from build123d import *

# Parameters (mm, degrees)
F0_R     = 8.25
F1_DEPTH = 2.5
F2_DEPTH = 2


with BuildPart() as f1:
    # F0 (on Top) → F1 (new body)
    with BuildSketch(Plane.XY):
        with BuildLine():
            ThreePointArc((32.0688115177, 8.9962420553), (27.6273312583, -1.0959733646), (33.9415177003, -10.1353654102))
            ThreePointArc((33.9415177003, -10.1353654102), (44.8086587224, -9.5259748044), (50.073819207, 0))
            ThreePointArc((50.073819207, 0), (43.8521719937, 10.0637054931), (32.0688115177, 8.9962420553))
        make_face()
        with Locations((38.823819207, 0)):
            Circle(F0_R, mode=Mode.SUBTRACT)
    extrude(amount=F1_DEPTH)



with BuildPart() as f1b:
    # F0 (on Top) → F1, piece 2 (new body)
    with BuildSketch(Plane.XY):
        with BuildLine():
            ThreePointArc((-45.6604546957, -2.0769858561), (-38.7231383621, 8.1832988366), (-29.426180793, 0))
            ThreePointArc((-29.426180793, 0), (-29.8634270645, -2.6501658772), (-31.1288181692, -5.0194165669))
            ThreePointArc((-31.1288181692, -5.0194165669), (-31.2694247122, -5.1976895367), (-31.4148838182, -5.3720257066))
            add(Edge.make_bspline(
                [(-29.035736161, -7.2045275043), (-30.5396230029, -7.95646964), (-32.2793337143, -6.7201835537), (-31.4148838182, -5.3720257066)],
                knots=[0, 0, 0, 0, 2.7840168374, 2.7840168374, 2.7840168374, 2.7840168374], degree=3))
            ThreePointArc((-29.035736161, -7.2045275043), (-27.0986692211, -3.8312855473), (-26.426180793, 0))
            ThreePointArc((-26.426180793, 0), (-27.6571196172, 5.1167287553), (-31.080565354, 9.1137454968))
            ThreePointArc((-31.080565354, 9.1137454968), (-44.3248746058, 9.0750961749), (-48.354220505, -3.5414640914))
            add(Edge.make_bspline(
                [(-45.6604546957, -2.0769858561), (-46.4311366211, -5.0662274962), (-47.7208728718, -5.0662274962), (-48.354220505, -3.5414640914)],
                knots=[0, 0, 0, 0, 3.0661165562, 3.0661165562, 3.0661165562, 3.0661165562], degree=3))
        make_face()
    extrude(amount=F1_DEPTH)


with BuildPart() as f1_1:
    add(f1.part)

    add(f1b.part)  # F2 merges F1b
    # F0 (on Top) → F2 (join)
    with BuildSketch(Plane.XY):
        with BuildLine():
            ThreePointArc((-26.426180793, 0), (-27.0986692211, -3.8312855473), (-29.035736161, -7.2045275043))
            add(Edge.make_bspline(
                [(-29.035736161, -7.2045275043), (-3.4389084727, 0), (5.4949232749, 0), (33.9415177003, -10.1353654102)],
                knots=[0, 0, 0, 0, 63.0454147004, 63.0454147004, 63.0454147004, 63.0454147004], degree=3))
            ThreePointArc((33.9415177003, -10.1353654102), (27.6273312583, -1.0959733646), (32.0688115177, 8.9962420553))
            add(Edge.make_bspline(
                [(-31.080565354, 9.1137454968), (-3.4389084727, 0), (5.4949232749, 0), (32.0688115177, 8.9962420553)],
                knots=[0, 0, 0, 0, 63.1494861922, 63.1494861922, 63.1494861922, 63.1494861922], degree=3))
            ThreePointArc((-31.080565354, 9.1137454968), (-27.6571196172, 5.1167287553), (-26.426180793, 0))
        make_face()
    extrude(amount=F2_DEPTH)


solid = f1_1.part
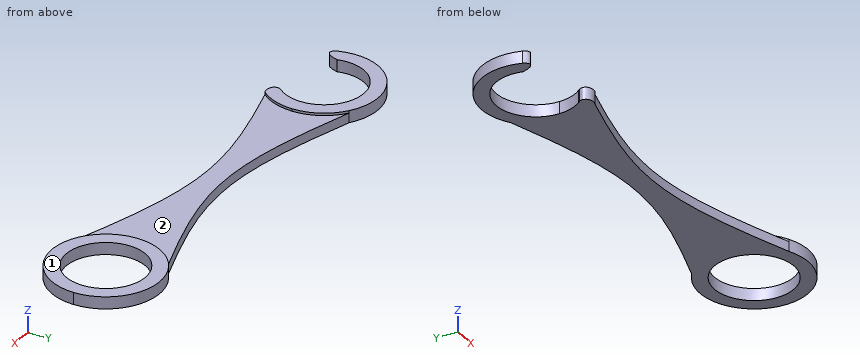
The model under review builds one solid part; all positions refer to its coordinate system, in mm. Face numbers are marked on the shaded views. Round coordinates to 2 decimals unless told otherwise and drop trailing zeros. Write each loop counter-clockwise with the first axis right and the second up, starting at its lowest first coordinate (ties: lowest second). Pieces come first, ordered by that corner, then holes. Notation, with made-up numbers: M 40,17.5 L 80,17.5 A23 cw 80,52.5 Z; hole C 0,36.25 d6. An arc over 180 degrees is marked long. Use a Markdown table: item, result. Add a question column.
Q1. We need section B-B, the plane x = -42. State the section outline as (y, z) points, plus the area to 3 significant figures.
Q2. To check wall thickness, follow line 1 (X direction, y = 0.5, z = 2.15); line 2 (X direction, y = 1.5, z = 1.9); line 3 (Y direction, x = 0.5, z = 0.85). State the ranges of each line that lie inside material, in increasing order.
Q3. Insertion check: pin 1 (6 mm diameter, centred on x = -2.5, y = -5, fed in from +Z); pin 2 (1.5 mm diameter, centred on y = 1, z = 0.5, fed in from -X); pin 3 (1 mm diameter, centred on x = 7, z = 0.5, fed in from -Y). Each pin has a flat end and moves straight along its axis. Give the tip position at first contact, or say it passes through.
Q4. The part is to be moulded in two halves that separate along X. For the marked faces 1 and 2, say which applies: pulls with the +X half, pulls with the -X half, needs draft (parallel to the pull), parting line crosses it, or undercut.
Q5. We need section A-A, the plane y = 5.5. Count the separate pieces of the cut face and the enclosed holes in it, plus the area to 3 significant figures.
Findings below:
| question | item | result |
|---|---|---|
| 1 | outline | M 7.03,0 L 10.39,0 L 10.39,2.5 L 7.03,2.5 Z |
| 1 | area | 8.40 mm² |
| 2 | line 1 | x = -48.92 to -45.91, -29.44 to -26.44, 27.58 to 30.59, 47.06 to 50.06 |
| 2 | line 2 | x = -48.83 to -45.79, -29.56 to 30.71, 46.94 to 49.97 |
| 2 | line 3 | y = -2.14 to 2.27 |
| 3 | pin 1 | stops at z = 2 |
| 3 | pin 2 | stops at x = -48.92 |
| 3 | pin 3 | stops at y = -2.74 |
| 4 | face 1 | needs draft |
| 4 | face 2 | undercut |
| 5 | separate pieces | 4 |
| 5 | enclosed holes | 0 |
| 5 | area | 69.8 mm² |
